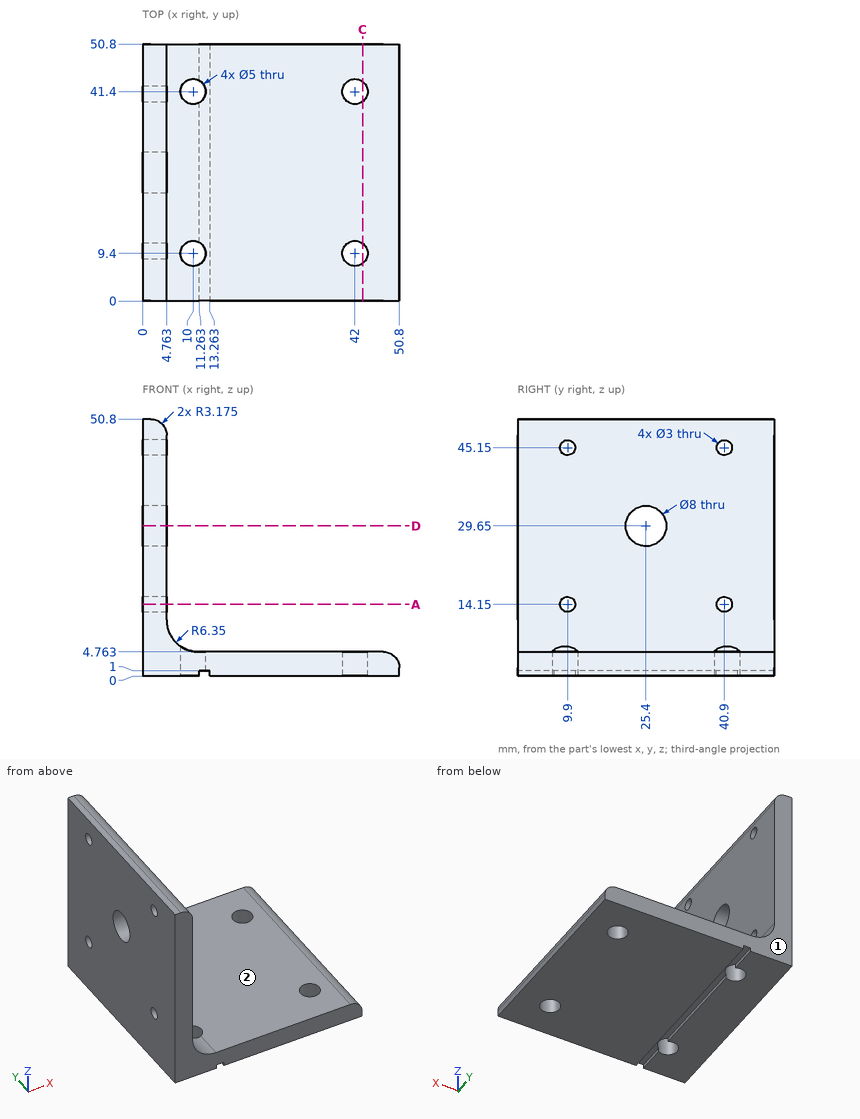
The figure shows three views and two pictorial views of one solid part (mm, origin at its lowest corner). Answer the questions. A direction names the side the tool comes from. Give positions to 0.01 mm unless a question says otherwise; leave off trailing zeros. Write each loop counter-clockwise with the first axis right and the second up, starting at its lowest first coordinate (ties: lowest second). Pieces come first, ordered by that corner, then holes. Notation, with made-up numbers: M 40,-2.75 L 82,-2.75 A21 ccw 82,32.25 Z; hole C -29,-7.5 d10. An arc over 180 degrees is marked long. One line per item, written item: value. Start each with the question number.
(1) Find section C-C (x = 43.5). Determine the outline of the cut face in (y, z).
(2) A tool of negligible diameter and unlimited length cuts with its end or side. For the marked faces 1 and 2, from which of +Z, -Z, +X, -X, +Y, -Y can it reach the whole face along a straight path? Write none if from no direction.
(3) Find the intervals of material crossed by line 1 (Y direction, x = 1, z = 14); line 2 (Z direction, x = 12.5, y = 34.5); line 3 (Z direction, x = 45.5, y = 25), in increasing order.
(4) Find section A-A (z = 14.15). Determine the outline of the cut face in (x, y), plus the area to 3 significant figures.
(5) Flat-ended cylindrical pins translate along their axes: pin 1 Ø1 at (x, y) = (12, 34.5) entering from -Z; pin 2 Ø2 at (y, z) = (32.5, 27.5) entering from +X; pin 3 Ø12 at (x, z) = (6, 17) entering from -Y; pin 4 Ø12 at (y, z) = (7.5, 13.5) entering from +X. Find the tip coordinate at first contact, or state that the pin passes through.
(6) Find section D-D (z = 29.65). Determine the outline of the cut face in (x, y), plus the area to 3 significant figures.
Results below:
1. outline: M 0,0 L 7.4,0 L 7.4,4.76 L 0,4.76 Z; M 11.4,0 L 39.4,0 L 39.4,4.76 L 11.4,4.76 Z; M 43.4,0 L 50.8,0 L 50.8,4.76 L 43.4,4.76 Z
2. face 1: +Z, -Z, +X, -X, +Y
2. face 2: +Z, +X, +Y, -Y
3. line 1: y = 0 to 8.41, 11.39 to 39.41, 42.39 to 50.8
3. line 2: z = 1 to 4.76
3. line 3: z = 0 to 4.76
4. outline: M 0,0 L 4.76,0 L 4.76,8.4 L 0,8.4 Z; M 0,11.4 L 4.76,11.4 L 4.76,39.4 L 0,39.4 Z; M 0,42.4 L 4.76,42.4 L 4.76,50.8 L 0,50.8 Z
4. area: 213 mm^2
5. pin 1: stops at z = 1
5. pin 2: stops at x = 4.76
5. pin 3: stops at y = 0
5. pin 4: stops at x = 5.89
6. outline: M 0,0 L 4.76,0 L 4.76,21.4 L 0,21.4 Z; M 0,29.4 L 4.76,29.4 L 4.76,50.8 L 0,50.8 Z
6. area: 204 mm^2
